from build123d import *

# Parameters (mm, degrees)
SKETCH1_R               = 75
BOSS_EXTRUDE1_DEPTH     = 35
CUT_EXTRUDE1_DEPTH      = 112.691539518
CUT_EXTRUDE1_DEPTH_BACK = 112.691539518
SKETCH2_R               = 2.38125
FILLET1_R               = 12.5
SKETCH3_R               = 5.953125
CUT_EXTRUDE2_DEPTH      = 6.35


with BuildPart() as part:
    # Sketch1 → Boss-Extrude1 (new body)
    with BuildSketch(Plane.XY):
        Circle(SKETCH1_R)
    extrude(amount=BOSS_EXTRUDE1_DEPTH)

    # Sketch2 → Cut-Extrude1 (cut, two sides: drawn at the far end of the back side and taken through both)
    with BuildSketch(Plane(origin=(0, 0, 0), x_dir=(1, 0, 0), z_dir=(0, 1, 0)).offset(-CUT_EXTRUDE1_DEPTH_BACK)):
        with Locations(Location((-6.045, -17.5, 0), (0, 0, 270))):
            Circle(SKETCH2_R)
        with Locations(Location((6.045, -17.5, 0), (0, 0, 270))):
            Circle(SKETCH2_R)
    extrude(amount=CUT_EXTRUDE1_DEPTH + CUT_EXTRUDE1_DEPTH_BACK, mode=Mode.SUBTRACT)

    # Fillet1
    fillet1_edges = [part.edges().sort_by_distance(p)[0] for p in [
        (-75, 0, 0),
        (-75, 0, 35),
    ]]
    fillet(fillet1_edges, radius=FILLET1_R)

    # Sketch3 → Cut-Extrude2 (cut)
    with BuildSketch(Plane(origin=(0, 75, 0), x_dir=(1, 0, 0), z_dir=(0, 1, 0))):
        with Locations(Location((-6.045, -17.5, 0), (0, 0, 270))):
            Circle(SKETCH3_R)
        with Locations(Location((6.045, -17.5, 0), (0, 0, 270))):
            Circle(SKETCH3_R)
    extrude(amount=-CUT_EXTRUDE2_DEPTH, mode=Mode.SUBTRACT)


solid = part.part
Verification items for the finished model (mm, model axes). A direction names the side the tool comes from. Coordinates: 2 decimals unless noted, no trailing zeros. Write each loop counter-clockwise with the first axis right and the second up, starting at its lowest first coordinate (ties: lowest second). Pieces come first, ordered by that corner, then holes. Notation, with made-up numbers: (45.5, 30) -> (69.5, 30) arc R24 ccw to (69.5, 49) -> close; hole circle Ø8 at (51, -36.75). An arc over 180 degrees is marked (long way). One line per item, written item: value. Start each with the question number.
Q1. Access from +Z, -Z, +X, -X, +Y, -Y to the whole of each face (thin tool, end or side, straight path). Record for faces 1 (the cylindrical face through (0.233, 71.869, 16.209)), 2 (the cylindrical face through (6.76, -4.14, 19.77)).
Q2. Mould release check, pull along X, two halves, no side actions. Record for faces 3 (the flat face through (-6, 68.65, 20.1)), 4 (the flat face through (-1, 1, 0)), 5 (the cylindrical face through (-3.168, -74.933, 17.43)): pulls with the +X half, pulls with the -X half, needs draft (parallel to the pull), parting line crosses it, or undercut.
Q3. Go/stop test with flat-tipped pins: P1, Ø6, axis at x = -45.5, z = 23, coming from the +Y side; P2, Ø3.5, axis at x = -8, z = 17.5, coming from the +Y side; P3, Ø1, axis at y = 55, z = 29.5, coming from the +X side. Record where each tip stops, or that it passes through.
Q4. Cross-section at C-C on z = 7. Enter the section's corners in (x, y).
Q5. Thickness scan on L1, parallel to X at y = -6, z = 17; L2, parallel to X at y = 4, z = 18; L3, parallel to X at y = 43, z = 33. Record the ranges inside material, lowest first. Write a range as from..to.
Q6. Cross-section at B-B on z = 17. Enter the section's corners in (x, y).
Q7. Cross-section at A-A on y = 0. Enter the section's corners in (x, z) (1 decimal), and give its area (3 significant figures).
Q8. Cross-section at D-D on y = 30. State how many separate pieces and enclosed holes the cut face has, and give its area (3 significant figures).
Checked values:
1. face 1: +Y
1. face 2: +Y, -Y
2. face 3: undercut
2. face 4: needs draft
2. face 5: parting line crosses it
3. P1: stops at y = 61.79
3. P2: stops at y = 68.65
3. P3: stops at x = 48.54
4. outline: circle Ø147.45 at (0, 0)
5. L1: x = -74.76..-8.37, -3.72..3.72, 8.37..74.76
5. L2: x = -74.89..-8.37, -3.72..3.72, 8.37..74.89
5. L3: x = -54.32..54.32
6. outline: (-11.98, 68.65) -> (-11.98, 74.04) arc R75 ccw to (-8.37, -74.53) -> (-8.37, 68.65) -> close; (-3.72, -74.91) arc R75 ccw to (3.72, -74.91) -> (3.72, 68.65) -> (0.11, 68.65) -> (0.11, 75) arc R75 ccw to (-0.11, 75) -> (-0.11, 68.65) -> (-3.72, 68.65) -> close; (8.37, -74.53) arc R75 ccw to (11.98, 74.04) -> (11.98, 68.65) -> (8.37, 68.65) -> close
7. outline: (-75, 12.5) arc R12.5 ccw to (-62.5, 0) -> (62.5, 0) arc R12.5 ccw to (75, 12.5) -> (75, 22.5) arc R12.5 ccw to (62.5, 35) -> (-62.5, 35) arc R12.5 ccw to (-75, 22.5) -> close; hole circle Ø4.8 at (-6, 17.5); hole circle Ø4.8 at (6, 17.5)
7. area: 5,080 mm²
8. separate pieces: 1
8. enclosed holes: 2
8. area: 4,630 mm²
